Autodesk Inventor part; units mm, degrees
ref_plane "YZ Plane" through (0, 0, 0) normal (1, 0, 0) x (0, 1, 0)
ref_plane "XZ Plane" through (0, 0, 0) normal (0, 1, 0) x (-1, 0, 0)
ref_plane "XY Plane" through (0, 0, 0) normal (0, 0, 1) x (1, 0, 0)
sketch "Sketch1" plane through (0, 0, 0) normal (0, 1, 0) x (-1, 0, 0)
  line L0 (0, 0) -> (-70, 0)
  line L1 (-70, 0) -> (-70, -76)
  line L2 (-70, -76) -> (0, -76)
  line L3 (0, -76) -> (0, 0)
  dimension "d0" = 70
  dimension "d1" = 76
extrude "Extrusion1" add sketch "Sketch1" along normal blind 3
sketch "Sketch2" plane through (0, 3, 0) normal (0, 1, 0) x (1, 0, 0)
  line L0 (70, 76) -> (0, 76)
  line L1 (16.33, 76) -> (30.05, 76)
  line L2 (30.05, 76) -> (30.05, 73)
  line L3 (30.05, 73) -> (16.33, 73)
  line L4 (16.33, 73) -> (16.33, 76)
  line L5 (39.95, 76) -> (53.67, 76)
  line L6 (53.67, 76) -> (53.67, 73)
  line L7 (53.67, 73) -> (39.95, 73)
  line L8 (39.95, 73) -> (39.95, 76)
  line L9 (30.05, 74.5) -> (39.95, 74.5) construction
  line L10 (0, 76) -> (0, 0)
  point P0 (23.19, 73)
  point P1 (46.81, 73)
  point P2 (35, 74.5)
  point P3 (35, 76)
  dimension "d4" = 13.72
  dimension "d5" = 13.72
  dimension "d6" = 3
  dimension "d29" = 16.33
extrude "Extrusion2" add sketch "Sketch2" along normal blind 6.3
sketch "Sketch3" plane through (0, 3, 0) normal (0, 1, 0) x (1, 0, 0)
  line L0 (0, 0) -> (70, 0)
  line L1 (44.67, 0) -> (53.67, 0)
  line L2 (53.67, 0) -> (53.67, 3)
  line L3 (53.67, 3) -> (44.67, 3)
  line L4 (44.67, 3) -> (44.67, 0)
  line L5 (53.67, 76) -> (53.67, 73)
  dimension "d10" = 9
  dimension "d11" = 3
extrude "Extrusion3" add sketch "Sketch3" along normal blind 7.1
sketch "Sketch4" plane through (0, 3, 0) normal (0, 1, 0) x (1, 0, 0)
  line L0 (16.33, 73) -> (16.33, 76)
  line L1 (0, 0) -> (44.67, 0)
  line L2 (44.67, 0) -> (44.67, 3)
  line L3 (12.87, 0) -> (28.97, 0)
  line L4 (28.97, 0) -> (28.97, 3)
  line L5 (28.97, 3) -> (12.87, 3)
  line L6 (12.87, 3) -> (12.87, 0)
  dimension "d16" = 16.1
  dimension "d17" = 15.7
extrude "Extrusion4" add sketch "Sketch4" along normal blind 6.2
sketch "Sketch5" plane through (0, 0, 0) normal (0, -1, 0) x (1, 0, 0)
  line L0 (0, 0) -> (70, 0)
  line L1 (0, -76) -> (0, 0)
  line L2 (4.5, -10) -> (65.5, -10) construction
  line L3 (65.5, -10) -> (65.5, -66) construction
  line L4 (65.5, -66) -> (4.5, -66) construction
  line L5 (4.5, -66) -> (4.5, -10) construction
  point P0 (35, -10)
  point P1 (35, 0)
  point P2 (4.5, -38)
  point P3 (0, -38)
  dimension "d20" = 10
  dimension "d21" = 4.5
hole "Hole1" at (4.5, 0, -10) at (4.5, 0, -66) at (65.5, 0, -66) at (65.5, 0, -10) direction (0, 1, 0) diameter 3.2 end through all counterbore diameter 6 counterbore depth 1
fillet "Fillet1" radius 6 4 edges at (0, 1.5, 0) (70, 1.5, 0) (70, 1.5, -76) (0, 1.5, -76)
sketch "Sketch6" plane through (0, 3, 0) normal (0, 1, 0) x (1, 0, 0)
  line L0 (16.33, 76) -> (6, 76)
  line L1 (13.03, 69.24) -> (56.97, 69.24) construction
  line L2 (0, 70) -> (70, 70) construction
  line L3 (13.03, 69.24) -> (13.03, 6.76) construction
  line L4 (6, 76) -> (6, 0) construction
  line L5 (37.62, 53.42) -> (37.62, 44.42)
  line L6 (31.62, 44.42) -> (31.62, 53.42)
  line L7 (33.37, 56.42) -> (35.87, 56.42)
  line L8 (35.87, 41.42) -> (33.37, 41.42)
  line L9 (31.62, 53.42) -> (33.37, 53.42)
  line L10 (35.87, 53.42) -> (37.62, 53.42)
  line L11 (37.62, 44.42) -> (35.87, 44.42)
  line L12 (33.37, 44.42) -> (31.62, 44.42)
  line L13 (33.37, 41.42) -> (33.37, 44.42)
  line L14 (33.37, 53.42) -> (33.37, 56.42)
  line L15 (35.87, 56.42) -> (35.87, 53.42)
  line L16 (35.87, 44.42) -> (35.87, 41.42)
  circle A0 centre (35.13, 61.87) radius 1.5
  point P0 (0, 0)
  point P1 (35, 69.24)
  point P2 (35, 70)
  point P3 (6, 38)
  point P4 (13.03, 38)
  point P5 (34.62, 56.42)
  point P6 (31.62, 48.92)
  dimension "d31" = 43.94
  dimension "d32" = 62.48
  dimension "d33" = 6
  dimension "d34" = 9
  dimension "d35" = 2.5
  dimension "d36" = 15
  dimension "d38" = 20.32
  dimension "d39" = 3
  dimension "d40" = 7.37
  dimension "d44" = 21.84
  dimension "d45" = 22.35
extrude "Extrusion5" cut sketch "Sketch6" against normal through all
fillet "Fillet2" radius 0.5 12 edges at (35.87, 1.5, -53.42) (33.37, 1.5, -53.42) (35.87, 1.5, -56.42) (33.37, 1.5, -56.42) (37.62, 1.5, -53.42) (37.62, 1.5, -44.42) (35.87, 1.5, -44.42) (35.87, 1.5, -41.42) (33.37, 1.5, -41.42) (33.37, 1.5, -44.42) (31.62, 1.5, -44.42) (31.62, 1.5, -53.42)
chamfer "Chamfer1" distance 2.5 angle 45 1 edges at (33.63, 3, -61.87)
sketch "Sketch7" plane through (30.05, 9.3, -76) normal (0, 0, -1) x (-1, 0, 0)
  line L0 (-9.9, -6.3) -> (-9.9, 0)
  line L1 (-23.62, 0) -> (-9.9, 0)
  line L2 (-33.95, -6.3) -> (-23.62, -6.3)
  line L3 (-23.62, 0) -> (-23.12, 0)
  line L4 (-23.12, 0) -> (-23.12, -6.3)
  line L5 (-23.12, -6.3) -> (-23.62, -6.3)
  line L6 (-23.62, -6.3) -> (-23.62, 0)
  line L7 (-10.4, 0) -> (-9.9, 0)
  line L8 (-9.9, 0) -> (-9.9, -6.3)
  line L9 (-9.9, -6.3) -> (-10.4, -6.3)
  line L10 (-10.4, -6.3) -> (-10.4, 0)
  line L11 (0, 0) -> (0.5, 0)
  line L12 (0.5, 0) -> (0.5, -6.3)
  line L13 (0.5, -6.3) -> (0, -6.3)
  line L14 (0, -6.3) -> (0, 0)
  line L15 (13.72, 0) -> (13.22, 0)
  line L16 (13.22, 0) -> (13.22, -6.3)
  line L17 (13.22, -6.3) -> (13.72, -6.3)
  line L18 (13.72, -6.3) -> (13.72, 0)
  point P0 (30.05, -9.3)
  dimension "d50" = 0.5
extrude "Extrusion6" cut sketch "Sketch7" against normal up to surface (3 mm away)
sketch "Sketch8" plane through (0, 3, 0) normal (0, 1, 0) x (1, 0, 0)
  line L0 (12.87, 3) -> (28.97, 3)
  line L1 (44.67, 0) -> (44.67, 3)
  line L2 (44.67, 3) -> (53.67, 3)
  line L3 (53.17, 73) -> (40.45, 73)
  line L4 (29.55, 73) -> (16.83, 73)
  line L5 (33.37, 41.92) -> (33.37, 43.92)
  line L6 (28.97, 3) -> (28.97, 3.2)
  line L7 (28.97, 3.2) -> (44.67, 3.2)
  line L8 (44.67, 3.2) -> (44.67, 3)
  line L9 (28.97, 3) -> (25.97, 3)
  line L10 (25.97, 3) -> (25.97, 6.2)
  line L11 (25.97, 6.2) -> (47.67, 6.2)
  line L12 (47.67, 6.2) -> (47.67, 3)
  line L13 (47.67, 3) -> (44.67, 3)
  line L14 (29.55, 73) -> (29.55, 72.8)
  line L15 (29.55, 72.8) -> (40.45, 72.8)
  line L16 (40.45, 72.8) -> (40.45, 73)
  line L17 (40.45, 73) -> (43.45, 73)
  line L18 (43.45, 73) -> (43.45, 69.8)
  line L19 (43.45, 69.8) -> (26.55, 69.8)
  line L20 (26.55, 69.8) -> (26.55, 73)
  line L21 (26.55, 73) -> (29.55, 73)
  point P0 (0, 0)
  dimension "d53" = 0.2
  dimension "d54" = 3
  dimension "d55" = 3
  dimension "d56" = 3
  dimension "d57" = 3
  dimension "d58" = 3
  dimension "d59" = 3
extrude "Extrusion7" add sketch "Sketch8" along normal up to surface (6.3 mm away)
fillet "Fillet3" radius 0.5 4 edges at (29.55, 6.15, -72.8) (40.45, 6.15, -72.8) (44.67, 6.15, -3.2) (28.97, 6.15, -3.2)
fillet "Fillet4" radius 1 8 edges at (43.45, 6.15, -73) (43.45, 6.15, -69.8) (26.55, 6.15, -73) (26.55, 6.15, -69.8) (47.67, 6.15, -3) (47.67, 6.15, -6.2) (25.97, 6.1, -3) (25.97, 6.15, -6.2)
equation "\"d5\" = d4"
equation "\"d55\" = d54"
equation "\"d56\" = d55"
equation "\"d57\" = d54"
equation "\"d58\" = d57"
equation "\"d59\" = d57"
properties part number "top"
Can you work these out from the model? Positions are in its coordinate system, mm. A direction names the side the tool comes from. Round coordinates to 2 decimals unless told otherwise and drop trailing zeros. Write each loop counter-clockwise with the first axis right and the second up, starting at its lowest first coordinate (ties: lowest second). Pieces come first, ordered by that corner, then holes. Notation, with made-up numbers: (28, 55) -> (50, 55) arc R10 cw to (50, 62) -> close; hole circle Ø5 at (-1, 16). An arc over 180 degrees is marked (long way). Use one line per item in the form item = value. Start each with the question number.
Q1. Imagine slicing it at A-A (z = -61.87). Please give me the cut outline in (x, y).
Q2. Which directions (+Z, -Z, +X, -X, +Y, -Y) give clear straight access to the entire face, cutting with the end or side of a thin tool? Please do faces 4 (the face through (4.4, 0.5, -63)), 5 (the face through (25.97, 6, -5)), 6 (the face through (33.37, 2, -55)), 7 (the face through (53.17, 6, -75)), 8 (the face through (49, 6, -73)).
Q3. Imagine slicing it at C-C (z = -50.5). Please give me the cut outline in (x, y), then the cut area to 3 significant figures.
Q4. If I drill on probe 1 along X at (y, z) = (2.3, -66); probe 2 along Z at (x, y) = (35.13, 0.35); probe 3 along X at (y, z) = (0.5, -66), over which ranges is the centre line in solid material (lowest first)? Write a range as [from, to].
Q5. We'd pull the mould along Z, two halves only. Please class faces 1 (the face through (37, 6, -6.2)), 2 (the face through (68.289, 1.521, -74.196)), 3 (the face through (28.97, 6, -1)): +Z half, -Z half, draft (parallel to the pull), parting line (faces both ways), or undercut.
Q6. I'm going to push flat-ended pins straight in: P1, Ø12, axis at x = 19, z = -24, coming from the +Y side; P2, Ø3, axis at y = 5.5, z = -1.5, coming from the +X side; P3, Ø1.5, axis at y = 1.5, z = -60, coming from the -X side; P4, Ø3, axis at x = 30, z = -71.5, coming from the +Y side. Where does each tip first touch, or does it pass through?
Q7. Imagine slicing it at D-D (x = 65.5). Please give me the cut outline in (y, z).
Q8. Imagine slicing it at B-B (x = 19). Please give me the cut outline in (y, z), then the cut area to 4 significant figures.
Worked out:
q1.outline = (0, 0) -> (33.63, 0) -> (33.63, 0.5) -> (31.13, 3) -> (0, 3) -> close; (36.63, 0) -> (70, 0) -> (70, 3) -> (39.13, 3) -> (36.63, 0.5) -> close
q2.face_4 = -Y
q2.face_5 = -X, +Y
q2.face_6 = +Y, -Y
q2.face_7 = -Z, +X, +Y
q2.face_8 = +X, +Y
q3.outline = (0, 0) -> (31.62, 0) -> (31.62, 3) -> (0, 3) -> close; (37.62, 0) -> (70, 0) -> (70, 3) -> (37.62, 3) -> close
q3.area = 192 mm^2
q4.probe_1 = [0, 2.9], [6.1, 63.9], [67.1, 70]
q4.probe_2 = [-76, -63.37], [-60.37, -56.42], [-41.42, 0]
q4.probe_3 = [0, 1.5], [7.5, 62.5], [68.5, 70]
q5.face_1 = undercut
q5.face_2 = -Z half
q5.face_3 = draft
q6.P1 = 3
q6.P2 = 53.67
q6.P3 = 0
q6.P4 = 9.3
q7.outline = (0, -75.81) -> (3, -75.81) -> (3, -67.6) -> (1, -67.6) -> (1, -69) -> (0, -69) -> close; (0, -63) -> (1, -63) -> (1, -64.4) -> (3, -64.4) -> (3, -11.6) -> (1, -11.6) -> (1, -13) -> (0, -13) -> close; (0, -7) -> (1, -7) -> (1, -8.4) -> (3, -8.4) -> (3, -0.19) -> (0, -0.19) -> close
q8.outline = (0, -76) -> (9.3, -76) -> (9.3, -73) -> (3, -73) -> (3, -3) -> (9.2, -3) -> (9.2, 0) -> (0, 0) -> close
q8.area = 265.5 mm^2
